Job drawing, mm, ordinate dimensions from the low corner. One solid piece. Give positions to 0.01 mm unless a question says otherwise; leave off trailing zeros. Write each loop counter-clockwise with the first axis right and the second up, starting at its lowest first coordinate (ties: lowest second). Pieces come first, ordered by that corner, then holes. Notation, with made-up numbers: M 5,43 L 62,43 A13 cw 62,62 Z; hole C 14,13.25 d7. An arc over 180 degrees is marked long. Use a Markdown table: item, result.
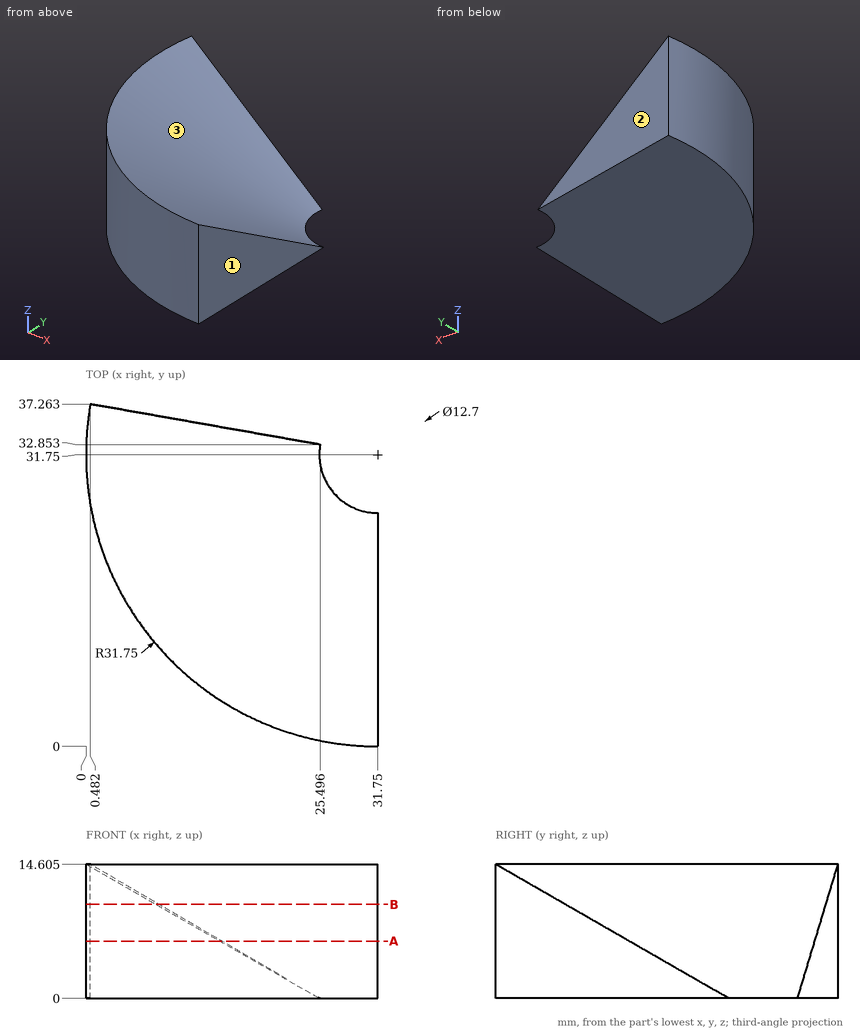
1. Drop flat-ended pins along their axis: P1, Ø1.5, axis at y = 24.5, z = 2, coming from the -X side; P2, Ø4, axis at x = 23.5, y = 29.5, coming from the +Z side (1 decimal); P3, Ø5, axis at x = 27, z = 9.5, coming from the +Y side. Give the stop position or say it passes through.
Findings below:
| item | result |
|---|---|
| P1 | x = 0.67 |
| P2 | z = 2.4 |
| P3 | y = 13.9 |
2. Cut at B-B, the plane z = 10.25. Give the cut face in (x, y), then the cut area to 3 significant figures.
Findings below:
| item | result |
|---|---|
| outline | M 0.48,37.26 A31.75 ccw 31.75,0 L 31.75,7.57 A24.18 cw 7.94,35.95 Z |
| area | 370 mm2 |
3. Cut at A-A, the plane z = 6.25. Give the cut face in (x, y).
Findings below:
| item | result |
|---|---|
| outline | M 0.48,37.26 A31.75 ccw 31.75,0 L 31.75,14.53 A17.22 cw 14.79,34.74 Z |
4. Drill centre lines: L1, parallel to X at y = 13, z = 5.25; L2, parallel to Z at x = 13, y = 33 (1 decimal); L3, parallel to Y at x = 28, z = 3.5 (1 decimal). Where is each one in solid material? Low to high.
Findings below:
| item | result |
|---|---|
| L1 | 6.13 to 31.75 |
| L2 | 0 to 7.2 |
| L3 | 0.2 to 19.9 |
5. Two-plate mould, pull along Y, no slides. Class the marked faces 1, 2 and 3: released by +Y, released by -Y, zero draft, split by the parting line, or undercut.
Findings below:
| item | result |
|---|---|
| face 1 | zero draft |
| face 2 | released by +Y |
| face 3 | undercut |
